Source: CAD feature listing. Evaluate the final solid. Frame: model axes, mm. A direction names the side the tool comes from. Coordinates: 2 decimals unless noted, no trailing zeros. Write each loop counter-clockwise with the first axis right and the second up, starting at its lowest first coordinate (ties: lowest second). Pieces come first, ordered by that corner, then holes. Notation, with made-up numbers: (85.5, 70.5) - (122.5, 70.5) arc R20 ccw to (122.5, 105.5) - close; hole circle Ø3 at (-29.5, 72.25). An arc over 180 degrees is marked (long way). One line per question, with ' | ' between items. Start each with the question number.
Q1. Line query: line 1 (X direction, y = 6, z = 1.5); line 2 (Z direction, x = 24, y = 13.5); line 3 (X direction, y = 18.5, z = 8.5). Output: solid intervals per line, ascending.
Q2. Cut plane A-A, the plane y = 4.75. Return loops of the section in (x, z).
Q3. Contact query for flat-ended pins moving along their axis: P1, Ø2, axis at x = 22.5, y = 5, coming from the +Z side; P2, Ø3, axis at x = 30, y = 17, coming from the +Z side; P3, Ø2, axis at y = 12, z = 11.5, coming from the +X side. Output: stop coordinate, or through.
Q4. Cut plane D-D, the plane y = 13.75. Return loops of the section in (x, z).
Q5. Cut plane B-B, the plane z = 9. Return loops of the section in (x, y), plus the area to 3 significant figures.
Q6. Cut plane C-C, the plane x = 30.5. Return loops of the section in (y, z), plus the area to 3 significant figures.
Q7. Access query for faces 1 (the face through (43, 16, 4)), 2 (the face through (12.314, 11, 17)), 3 (the face through (38, 10, 4)). Directions: +Z, -Z, +X, -X, +Y, -Y. A direction counts if a zero-diameter tool reaches every point of the face in a straight line with its end or side. Return the directions, or none.
```python
from build123d import *

# Parameters (mm, degrees)
F1_DEPTH = 22.5
F2_W     = 10
F2_H     = 10
F3_DEPTH = 25


with BuildPart() as f1:
    # F0 (on Front) → F1 (new body)
    with BuildSketch(Plane.XZ):
        Polygon((0, 20), (0, 0), (43, 0), (43, 7.5), (24.230773, 7.5), (24.230773, 15), (12.313999, 15), (12.313999, 20), align=None)
    extrude(amount=-F1_DEPTH)

    # F2 (on face) → F3 (cut)
    with BuildSketch(Plane.XY.offset(7.5)):
        with Locations((38, 5)):
            Rectangle(F2_W, F2_H)
    extrude(amount=-F3_DEPTH, mode=Mode.SUBTRACT)


solid = f1.part
```
Reply:
1) line 1: x = 0 to 33 | line 2: z = 0 to 15 | line 3: x = 0 to 24.23
2) outline: (0, 0) - (33, 0) - (33, 7.5) - (24.23, 7.5) - (24.23, 15) - (12.31, 15) - (12.31, 20) - (0, 20) - close
3) P1: stops at z = 15 | P2: stops at z = 7.5 | P3: stops at x = 24.23
4) outline: (0, 0) - (43, 0) - (43, 7.5) - (24.23, 7.5) - (24.23, 15) - (12.31, 15) - (12.31, 20) - (0, 20) - close
5) outline: (0, 0) - (24.23, 0) - (24.23, 22.5) - (0, 22.5) - close | area: 545 mm^2
6) outline: (0, 0) - (22.5, 0) - (22.5, 7.5) - (0, 7.5) - close | area: 169 mm^2
7) face 1: +Z, -Z, +X, +Y, -Y | face 2: +Z, +X, +Y, -Y | face 3: +Z, -Z, +X, -Y
